```python
from build123d import *

# Parameters (mm, degrees)
CUT_EXTRUDE1_DEPTH = 4


with BuildPart() as part:
    # Sketch1 → Revolve1 (revolve)
    with BuildSketch(Plane(origin=(0, 0, 0), x_dir=(0, 0, -1), z_dir=(1, 0, 0))):
        Polygon((-5, 0), (-5, 3), (121.2, 3), (121.2, 8), (125.2, 8), (125.2, 0), align=None)
    revolve(axis=Axis((0, 0, -125.2), (0, 0, 1)))

    # Sketch2 → Revolve2 (revolve)
    with BuildSketch(Plane(origin=(0, 0, 0), x_dir=(0, 0, -1), z_dir=(1, 0, 0))):
        with BuildLine():
            Line((-21, 0), (-21, 2.3865))
            Line((-21, 2.3865), (-20.3865, 3))
            Line((-20.3865, 3), (-8.148486452, 3))
            Line((-8.148486452, 3), (-6.599415898, 2.436184428))
            ThreePointArc((-6.599415898, 2.436184428), (-6.498392718, 2.409115348), (-6.394203812, 2.4))
            Line((-6.394203812, 2.4), (-5.6, 2.4))
            ThreePointArc((-5.6, 2.4), (-5.175735931, 2.575735931), (-5, 3))
            Line((-5, 3), (-4, 3))
            Line((-4, 3), (-4, 0))
            Line((-4, 0), (-21, 0))
        make_face()
    revolve(axis=Axis((0, 0, 4), (0, 0, 1)))

    # Sketch3 → Cut-Extrude1 (cut)
    with BuildSketch(Plane.XY.offset(2)):
        Polygon((-5, 10), (-5, -5), (-2.5, -5), (-2.5, 5), (2.5, 5), (2.5, -5), (5, -5), (5, 10), align=None)
    extrude(amount=CUT_EXTRUDE1_DEPTH, mode=Mode.SUBTRACT)


solid = part.part
```
The model under review builds one solid part; all positions refer to its coordinate system, in mm. A direction names the side the tool comes from. Give positions to 0.01 mm unless a question says otherwise; leave off trailing zeros. Write each loop counter-clockwise with the first axis right and the second up, starting at its lowest first coordinate (ties: lowest second). Pieces come first, ordered by that corner, then holes.
(1) Consider section D-D, the plane x = 5.5. Give the boundary of the cut face in (y, z).
(2) The part is to be moulded in two halves that separate along Z. For faces 1 (the cylindrical face through (0, -3, 14)), 2 (the flat face through (2.5, 0, 4)), 3 (the flat face through (-0.1, -3.4, -121.2)), say which applies: released by +Z, released by -Z, zero draft, split by the parting line, or undercut.
(3) For P1, Ø3, axis at x = 4.5, y = -4, coming from the +Z side; P2, Ø1.5, axis at x = 2, z = -74, coming from the +Y side; P3, Ø2.5, axis at y = -0.5, z = 3, coming from the -X side, all flat-tipped, find the tip position at first contact; note any pin that passes through.
(4) Consider section C-C, the plane z = -51. Give the boundary of the cut face in (x, y), and give its area (3 significant figures).
(5) To check wall thickness, follow L1, parallel to Z at x = 5.5, y = 4; L2, parallel to Y at x = -0.5, z = -4.5; L3, parallel to Y at x = -2.5, z = -45. State the ranges of each line that lie inside material, in increasing order.
(6) Consider section B-B, the plane x = 0. Give the boundary of the cut face in (y, z), and give its area (3 significant figures).
(7) Consider section A-A, the plane y = 0. Give the boundary of the cut face in (x, z), and give its area (3 significant figures).
(8) Tool access review of faces 4 (the cylindrical face through (0, -3, -59)), 5 (the cylindrical face through (-2.024, 1.29, 5.992)), 6 (the flat face through (-2.5, 0, 4)): name each direction out of +Z, -Z, +X, -X, +Y, -Y from which nothing blocks a thin tool from reaching the whole face with its end or side.
Returned:
1. outline: (-5.81, -125.2) - (5.81, -125.2) - (5.81, -121.2) - (-5.81, -121.2) - close
2. face 1: zero draft
2. face 2: undercut
2. face 3: released by +Z
3. P1: stops at z = -121.2
3. P2: stops at y = 2.73
3. P3: stops at x = -3
4. outline: circle Ø6 at (0, 0)
4. area: 28.3 mm2
5. L1: z = -125.2 to -121.2
5. L2: y = -2.96 to 2.96
5. L3: y = -1.66 to 1.66
6. outline: (-8, -125.2) - (8, -125.2) - (8, -121.2) - (3, -121.2) - (3, 5) arc R0.6 cw to (2.4, 5.6) - (2.4, 6.39) arc R0.6 cw to (2.44, 6.6) - (3, 8.15) - (3, 20.39) - (2.39, 21) - (-2.39, 21) - (-3, 20.39) - (-3, 8.15) - (-2.44, 6.6) arc R0.6 cw to (-2.4, 6.39) - (-2.4, 5.6) arc R0.6 cw to (-3, 5) - (-3, -121.2) - (-8, -121.2) - close
6. area: 914 mm2
7. outline: (-8, -125.2) - (8, -125.2) - (8, -121.2) - (3, -121.2) - (3, 2) - (2.5, 2) - (2.5, 5.27) arc R0.6 cw to (2.4, 5.6) - (2.4, 6.39) arc R0.6 cw to (2.44, 6.6) - (3, 8.15) - (3, 20.39) - (2.39, 21) - (-2.39, 21) - (-3, 20.39) - (-3, 8.15) - (-2.44, 6.6) arc R0.6 cw to (-2.4, 6.39) - (-2.4, 5.6) arc R0.6 cw to (-2.5, 5.27) - (-2.5, 2) - (-3, 2) - (-3, -121.2) - (-8, -121.2) - close
7. area: 911 mm2
8. face 4: +Z
8. face 5: none
8. face 6: -X, +Y, -Y
